For this review, take the finished solid that the model builds, in its own axes (mm). Round coordinates to 2 decimals unless told otherwise and drop trailing zeros. Write each loop counter-clockwise with the first axis right and the second up, starting at its lowest first coordinate (ties: lowest second). Pieces come first, ordered by that corner, then holes. Notation, with made-up numbers: M -28.5,22 L 26.5,22 A11 ccw 26.5,37 Z; hole C 72,24.25 d11. An arc over 180 degrees is marked long. Write each question's results on one line, items separated by ' | '. Start each with the question number.
```python
from build123d import *

# Parameters (mm, degrees)
SKETCH2_W              = 500
SKETCH2_H              = 506
BOSS_EXTRUDE1_DEPTH    = 6
CUT_EXTRUDE1_DEPTH     = 6
LPATTERN1_COUNT        = 4
LPATTERN1_PITCH        = 111.1
LPATTERN2_COUNT        = 2
LPATTERN2_PITCH        = 188
LPATTERN3_COPY_1_DEPTH = 6
LPATTERN3_COPY_2_DEPTH = 6
LPATTERN3_COPY_3_DEPTH = 6
SKETCH9_W              = 28.3
SKETCH9_H              = 6
CUT_EXTRUDE3_DEPTH     = 3
LPATTERN5_COUNT        = 5
LPATTERN5_PITCH        = 111


with BuildPart() as part:
    # Sketch2 → Boss-Extrude1 (new body)
    with BuildSketch(Plane(origin=(0, 0, 0), x_dir=(1, 0, 0), z_dir=(0, 1, 0))):
        Rectangle(SKETCH2_W, SKETCH2_H)
    extrude(amount=BOSS_EXTRUDE1_DEPTH)

    # Sketch3 → Cut-Extrude1 (cut)
    with BuildSketch(Plane(origin=(0, 6, 0), x_dir=(1, 0, 0), z_dir=(0, 1, 0))):
        with BuildLine():
            add(Edge.make_bspline(
                [(194.4, 253), (194.2, 253), (194.2, 250), (194.2, 247), (194.4, 247)],
                knots=[3.141592654, 3.141592654, 3.141592654, 4.71238898, 4.71238898, 6.283185307, 6.283185307, 6.283185307], degree=2, weights=[1, 0.707106781, 1, 0.707106781, 1]))
            Line((194.4, 253), (138.8, 253))
            add(Edge.make_bspline(
                [(138.8, 247), (139, 247), (139, 250), (139, 253), (138.8, 253)],
                knots=[0, 0, 0, 1.570796327, 1.570796327, 3.141592654, 3.141592654, 3.141592654], degree=2, weights=[1, 0.707106781, 1, 0.707106781, 1]))
            Line((138.8, 247), (194.4, 247))
        make_face()
    cut_extrude1 = extrude(amount=-CUT_EXTRUDE1_DEPTH, mode=Mode.SUBTRACT)

    # LPattern1: Cut-Extrude1 ×4
    with Locations(*[(-i * LPATTERN1_PITCH, 0, 0) for i in range(1, LPATTERN1_COUNT)]):
        add(cut_extrude1, mode=Mode.SUBTRACT)

    # LPattern2: Cut-Extrude1 ×2
    with Locations(*[(0, 0, i * LPATTERN2_PITCH) for i in range(1, LPATTERN2_COUNT)]):
        add(cut_extrude1, mode=Mode.SUBTRACT)

    # LPattern3 copy 1 sketch → LPattern3 copy 1 (cut)
    with BuildSketch(Plane(origin=(-111.1, 6, 188), x_dir=(1, 0, 0), z_dir=(0, 1, 0))):
        with BuildLine():
            add(Edge.make_bspline(
                [(194.4, 253), (194.2, 253), (194.2, 250), (194.2, 247), (194.4, 247)],
                knots=[3.141592654, 3.141592654, 3.141592654, 4.71238898, 4.71238898, 6.283185307, 6.283185307, 6.283185307], degree=2, weights=[1, 0.707106781, 1, 0.707106781, 1]))
            Line((194.4, 253), (138.8, 253))
            add(Edge.make_bspline(
                [(138.8, 247), (139, 247), (139, 250), (139, 253), (138.8, 253)],
                knots=[0, 0, 0, 1.570796327, 1.570796327, 3.141592654, 3.141592654, 3.141592654], degree=2, weights=[1, 0.707106781, 1, 0.707106781, 1]))
            Line((138.8, 247), (194.4, 247))
        make_face()
    extrude(amount=-LPATTERN3_COPY_1_DEPTH, mode=Mode.SUBTRACT)

    # LPattern3 copy 2 sketch → LPattern3 copy 2 (cut)
    with BuildSketch(Plane(origin=(-222.2, 6, 188), x_dir=(1, 0, 0), z_dir=(0, 1, 0))):
        with BuildLine():
            add(Edge.make_bspline(
                [(194.4, 253), (194.2, 253), (194.2, 250), (194.2, 247), (194.4, 247)],
                knots=[3.141592654, 3.141592654, 3.141592654, 4.71238898, 4.71238898, 6.283185307, 6.283185307, 6.283185307], degree=2, weights=[1, 0.707106781, 1, 0.707106781, 1]))
            Line((194.4, 253), (138.8, 253))
            add(Edge.make_bspline(
                [(138.8, 247), (139, 247), (139, 250), (139, 253), (138.8, 253)],
                knots=[0, 0, 0, 1.570796327, 1.570796327, 3.141592654, 3.141592654, 3.141592654], degree=2, weights=[1, 0.707106781, 1, 0.707106781, 1]))
            Line((138.8, 247), (194.4, 247))
        make_face()
    extrude(amount=-LPATTERN3_COPY_2_DEPTH, mode=Mode.SUBTRACT)

    # LPattern3 copy 3 sketch → LPattern3 copy 3 (cut)
    with BuildSketch(Plane(origin=(-333.3, 6, 188), x_dir=(1, 0, 0), z_dir=(0, 1, 0))):
        with BuildLine():
            add(Edge.make_bspline(
                [(194.4, 253), (194.2, 253), (194.2, 250), (194.2, 247), (194.4, 247)],
                knots=[3.141592654, 3.141592654, 3.141592654, 4.71238898, 4.71238898, 6.283185307, 6.283185307, 6.283185307], degree=2, weights=[1, 0.707106781, 1, 0.707106781, 1]))
            Line((194.4, 253), (138.8, 253))
            add(Edge.make_bspline(
                [(138.8, 247), (139, 247), (139, 250), (139, 253), (138.8, 253)],
                knots=[0, 0, 0, 1.570796327, 1.570796327, 3.141592654, 3.141592654, 3.141592654], degree=2, weights=[1, 0.707106781, 1, 0.707106781, 1]))
            Line((138.8, 247), (194.4, 247))
        make_face()
    extrude(amount=-LPATTERN3_COPY_3_DEPTH, mode=Mode.SUBTRACT)

    # Sketch9 → Cut-Extrude3 (cut)
    with BuildSketch(Plane(origin=(0, 6, 0), x_dir=(1, 0, 0), z_dir=(0, 1, 0))):
        with Locations((222.2, 250)):
            Rectangle(SKETCH9_W, SKETCH9_H)
    cut_extrude3 = extrude(amount=-CUT_EXTRUDE3_DEPTH, mode=Mode.SUBTRACT)

    # LPattern5: Cut-Extrude3 ×5
    with Locations(*[(-i * LPATTERN5_PITCH, 0, 0) for i in range(1, LPATTERN5_COUNT)]):
        add(cut_extrude3, mode=Mode.SUBTRACT)


solid = part.part
```
Item 1: We need section A-A on x = 156.5. State the section outline as (y, z) points, then the cut area to 3 significant figures.
Item 2: Insertion check: P1, Ø1, axis at x = -152, y = 4, coming from the -Z side; P2, Ø6.5, axis at x = 111.5, z = -251.5, coming from the +Y side. Each pin has a flat end and moves straight along its axis. Give the tip position at first contact, or say it passes through.
Item 3: For probe 1 along Z at (x, y) = (68, 4.5); probe 2 along Z at (x, y) = (-118, 4.25), list the stretches that pass through material, from the lowest coordinate up.
Numbers:
1) outline: M 0,-247 L 6,-247 L 6,-65 L 0,-65 Z; M 0,-59 L 6,-59 L 6,253 L 0,253 Z | area: 2,960 mm^2
2) P1: stops at z = -247 | P2: stops at y = 3
3) probe 1: z = -247 to -65, -59 to 253 | probe 2: z = -247 to 253
